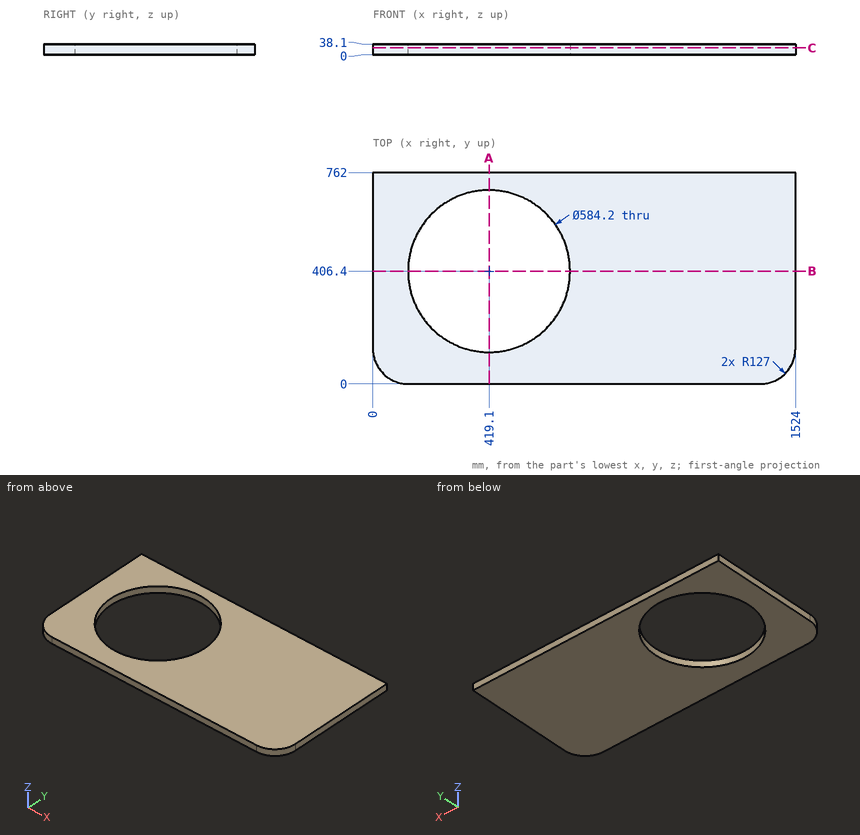
Input: dimensioned drawing with shaded views. Units: mm. Origin: part minimum x, y, z. Round coordinates to 2 decimals unless told otherwise and drop trailing zeros. Loops run counter-clockwise (first coordinate to the right, second up) from the corner with the lowest first, then second, coordinate; pieces in that order, holes last. Notation, with made-up numbers: M 36.5,85 L 93.5,85 A12 cw 93.5,106 Z; hole C 38,19 d6. An arc over 180 degrees is marked long. Answer in a Markdown table with one row per item. Add a question column.
1. Section B-B (y = 406.4). Output: boundary loops of the cut face in (x, z).
2. Ray query, probe 1 along Y at (x, z) = (419.1, 24); probe 2 along X at (y, z) = (406, 9); probe 3 along X at (y, z) = (209.5, 18.5). Return the intervals inside material, ascending.
3. Section A-A (x = 419.1). Output: boundary loops of the cut face in (y, z).
4. Section C-C (z = 24). Output: boundary loops of the cut face in (x, y).
Values follow:
| question | item | result |
|---|---|---|
| 1 | outline | M 0,0 L 127,0 L 127,38.1 L 0,38.1 Z; M 711.2,0 L 1524,0 L 1524,38.1 L 711.2,38.1 Z |
| 2 | probe 1 | 0 to 114.3, 698.5 to 762 |
| 2 | probe 2 | 0 to 127, 711.2 to 1524 |
| 2 | probe 3 | 0 to 203.34, 634.86 to 1524 |
| 3 | outline | M 0,0 L 114.3,0 L 114.3,38.1 L 0,38.1 Z; M 698.5,0 L 762,0 L 762,38.1 L 698.5,38.1 Z |
| 4 | outline | M 0,127 A127 ccw 127,0 L 1397,0 A127 ccw 1524,127 L 1524,762 L 0,762 Z; hole C 419.1,406.4 d584.2 |
